Geometry: final body of the model. Coordinates: model frame, mm. Face numbers are marked on the shaded views. A direction names the side the tool comes from. Give positions to 0.01 mm unless a question says otherwise; leave off trailing zeros. Write each loop counter-clockwise with the first axis right and the second up, starting at its lowest first coordinate (ties: lowest second). Pieces come first, ordered by that corner, then holes. Notation, with made-up numbers: M 34.25,88.5 L 65.25,88.5 A29 cw 65.25,123.5 Z; hole C 10,11 d4. An arc over 180 degrees is marked long. Use a Markdown table: item, result. Add a question column.
1) Section B-B on x = 123. Return the cut outline in (y, z), then the cut area to 3 significant figures.
2) Pin query (flat end, axial travel): pin 1 (10 mm diameter, centred on x = 160.5, z = 15, fed in from -Y); pin 2 (2.5 mm diameter, centred on x = 197.5, y = 20, fed in from -Z); pin 3 (12.5 mm diameter, centred on x = 125, y = 16.5, fed in from +Z); pin 4 (1.5 mm diameter, centred on x = 197, z = 15.5, fed in from -Y). Return the tip coordinate at first contact, or that it passes through.
3) Section A-A on y = 12.7. Return the cut outline in (x, z), then the cut area to 3 significant figures.
4) Set-up query: the marked faces 1 and 2. Return all of +Z, -Z, +X, -X, +Y, -Y with unobstructed straight access to the full face (end or side cutting, diameter ignored); none if empty.
5) Line query: line 1 (X direction, y = 13, z = 11.25); line 2 (Z direction, x = 12, y = 5.75); line 3 (Y direction, x = 201.5, z = 6.5). Output: solid intervals per line, ascending.
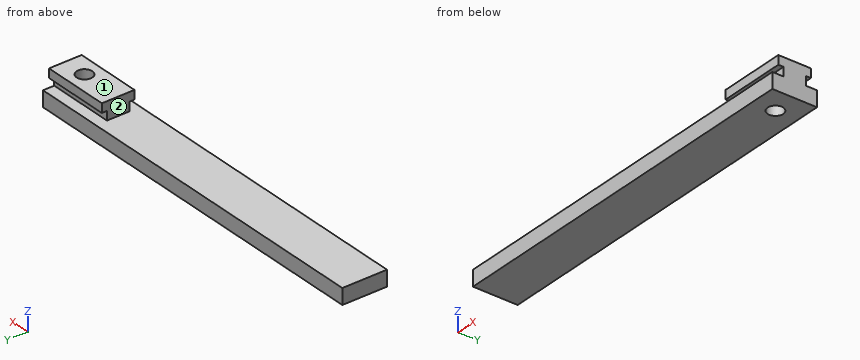
Autodesk Inventor part; units mm, degrees
ref_plane "YZ Plane" through (0, 0, 0) normal (1, 0, 0) x (0, 1, 0)
ref_plane "XZ Plane" through (0, 0, 0) normal (0, 1, 0) x (-1, 0, 0)
ref_plane "XY Plane" through (0, 0, 0) normal (0, 0, 1) x (1, 0, 0)
sketch "Sketch1" plane through (0, 0, 0) normal (0, 0, 1) x (1, 0, 0)
  line L0 (0, 0) -> (215.9, 0)
  line L1 (215.9, 0) -> (215.9, 25.4)
  line L2 (215.9, 25.4) -> (0, 25.4)
  line L3 (0, 25.4) -> (0, 0)
  dimension "d0" = 215.9
  dimension "d1" = 25.4
extrude "Extrusion1" add sketch "Sketch1" along normal blind 8.89
sketch "Sketch2" plane through (0, 0, 8.89) normal (0, 0, 1) x (1, 0, 0)
  line L0 (0, 0) -> (215.9, 0)
  line L1 (215.9, 0) -> (215.9, 25.4)
  line L2 (215.9, 25.4) -> (177.8, 25.4)
  line L3 (177.8, 25.4) -> (177.8, 0)
  line L4 (177.8, 0) -> (215.9, 0)
  line L5 (215.9, 0) -> (215.9, 25.4)
  line L6 (215.9, 25.4) -> (177.8, 25.4)
  line L7 (177.8, 25.4) -> (177.8, 12.7)
  line L8 (177.8, 12.7) -> (215.9, 12.7)
  line L9 (215.9, 12.7) -> (215.9, 25.4)
  line L10 (215.9, 25.4) -> (177.8, 25.4)
  line L11 (177.8, 25.4) -> (177.8, 19.05)
  line L12 (177.8, 19.05) -> (215.9, 19.05)
  line L13 (215.9, 19.05) -> (215.9, 25.4)
  line L14 (215.9, 0) -> (177.8, 0)
  line L15 (177.8, 0) -> (177.8, 6.35)
  line L16 (177.8, 6.35) -> (215.9, 6.35)
  line L17 (215.9, 6.35) -> (215.9, 0)
  dimension "d4" = 6.35
  dimension "d5" = 38.1
extrude "Extrusion2" add sketch "Sketch2" along normal blind 5.08 contours L3 L8 L1 L16 | L3 L12 L1 L8
sketch "Sketch3" plane through (0, 0, 13.97) normal (0, 0, 1) x (1, 0, 0)
  line L0 (215.9, 19.05) -> (177.8, 19.05)
  line L1 (177.8, 19.05) -> (177.8, 6.35)
  line L2 (177.8, 6.35) -> (215.9, 6.35)
  line L3 (215.9, 6.35) -> (215.9, 19.05)
  line L4 (215.9, 19.05) -> (177.8, 19.05)
  line L5 (177.8, 19.05) -> (177.8, 6.35)
  line L6 (215.9, 19.05) -> (177.8, 19.05)
  line L7 (177.8, 19.05) -> (177.8, 21.971)
  line L8 (177.8, 21.971) -> (215.9, 21.971)
  line L9 (215.9, 21.971) -> (215.9, 19.05)
  line L10 (215.9, 6.35) -> (177.8, 6.35)
  line L11 (177.8, 6.35) -> (177.8, 3.429)
  line L12 (177.8, 3.429) -> (215.9, 3.429)
  line L13 (215.9, 3.429) -> (215.9, 6.35)
  point P0 (0, 0)
  dimension "d8" = 2.921
  dimension "d9" = 2.921
extrude "Extrusion3" add sketch "Sketch3" along normal blind 5.08
sketch "Sketch4" plane through (0, 0, 0) normal (0, 0, -1) x (-1, 0, 0)
  circle A0 centre (-202.0681, 12.7) radius 4.445
  dimension "d12" = 8.89
extrude "Extrusion4" cut sketch "Sketch4" against normal blind 127
properties part number "Piece One-" material "Steel"
Found:
| question | item | result |
|---|---|---|
| 1 | outline | M 0,0 L 25.4,0 L 25.4,8.89 L 0,8.89 Z |
| 1 | area | 226 mm² |
| 2 | pin 1 | through |
| 2 | pin 2 | z = 0 |
| 2 | pin 3 | z = 8.89 |
| 2 | pin 4 | y = 3.43 |
| 3 | outline | M 0,0 L 197.62,0 L 197.62,19.05 L 177.8,19.05 L 177.8,8.89 L 0,8.89 Z; M 206.51,0 L 215.9,0 L 215.9,19.05 L 206.51,19.05 Z |
| 3 | area | 2,140 mm² |
| 4 | face 1 | +Z, +X, -X, +Y, -Y |
| 4 | face 2 | +Z, -X, +Y, -Y |
| 5 | line 1 | 177.8 to 197.63, 206.5 to 215.9 |
| 5 | line 2 | 0 to 8.89 |
| 5 | line 3 | 0 to 8.29, 17.11 to 25.4 |
